```python
from build123d import *

# Parameters (mm, degrees)
ESBO_O1_R                = 1.393053459
ESBO_O1_R_2              = 4
ESBO_O1_R_3              = 1.370583382
RESSALTO_EXTRUS_O1_DEPTH = 40
CORTE_EXTRUS_O1_START    = -26
ESBO_O5_R                = 1.393053459
ESBO_O5_R_2              = 1.370583382
CORTE_EXTRUS_O1_DEPTH    = 26
ESBO_O8_W                = 7
ESBO_O8_H                = 2


with BuildPart() as part:
    # Esboço1 → Ressalto-extrusão1 (new body)
    with BuildSketch(Plane.XY):
        with BuildLine():
            Line((-90, -22.423877672), (-90, -19))
            ThreePointArc((-90, -19), (-71, 0), (-90, 19))
            Line((-90, 19), (-90, 23.042521341))
            Line((-90, 23.042521341), (-72.401791427, 23.042521341))
            ThreePointArc((-72.401791427, 23.042521341), (-59.673869366, 17.770443402), (-54.401791427, 5.042521341))
            Line((-54.401791427, 5.042521341), (-54.401791427, -4.423877672))
            ThreePointArc((-54.401791427, -4.423877672), (-59.673869366, -17.151799733), (-72.401791427, -22.423877672))
            Line((-72.401791427, -22.423877672), (-90, -22.423877672))
        make_face()
        with Locations((-64.399704634, 15.948259466)):
            Circle(ESBO_O1_R, mode=Mode.SUBTRACT)
        with Locations((-61.189365531, 0)):
            Circle(ESBO_O1_R_2, mode=Mode.SUBTRACT)
        with Locations((-64.399704634, -14.228928105)):
            Circle(ESBO_O1_R_3, mode=Mode.SUBTRACT)
    extrude(amount=RESSALTO_EXTRUS_O1_DEPTH)

    # Esboço5 → Corte-extrusão1 (cut)
    # profile 1 of 3: a face of its own
    with BuildSketch(Plane.XY.offset(40).offset(CORTE_EXTRUS_O1_START)):
        with BuildLine():
            add(Edge.make_bspline(
                [(-54.401791427, 5.042521341), (-55.530001159, 10.383788665), (-70.453859237, 8.636772089), (-68.317241022, 19.151967947), (-69.419494496, 22.655429754), (-72.401791427, 23.042521341)],
                knots=[0, 0, 0, 0, 0.59841234, 0.778329044, 1, 1, 1, 1], degree=3))
            ThreePointArc((-72.401791427, 23.042521341), (-59.673869366, 17.770443402), (-54.401791427, 5.042521341))
        make_face()
        with Locations((-64.399704634, 15.948259466)):
            Circle(ESBO_O5_R, mode=Mode.SUBTRACT)
    # profile 2 of 3: a face of its own
    with BuildSketch(Plane.XY.offset(40).offset(CORTE_EXTRUS_O1_START)):
        with BuildLine():
            add(Edge.make_bspline(
                [(-54.455116699, -5.808387052), (-55.021642733, -6.906023952), (-60.824639792, -8.65742119), (-69.99744996, -12.030398314), (-68.624992944, -17.552582132), (-68.947451642, -20.712215011), (-69.65151808, -21.847158712), (-70.29295532, -22.299917789)],
                knots=[0.054307943, 0.054307943, 0.054307943, 0.054307943, 0.303140082, 0.59841234, 0.778329044, 0.849345989, 0.932732603, 0.932732603, 0.932732603, 0.932732603], degree=3))
            ThreePointArc((-70.29295532, -22.299917789), (-59.419167454, -16.891895749), (-54.455116699, -5.808387052))
        make_face()
        with Locations((-64.399704634, -14.228928105)):
            Circle(ESBO_O5_R_2, mode=Mode.SUBTRACT)
    # profile 3 of 3: a face of its own
    with BuildSketch(Plane.XY.offset(40).offset(CORTE_EXTRUS_O1_START)):
        with Locations((-64.399704634, 15.948259466)):
            Circle(ESBO_O5_R)
    extrude(amount=CORTE_EXTRUS_O1_DEPTH, mode=Mode.SUBTRACT)

    # Varredura de corte1: sweep along a path in Esboço7
    with BuildLine(Plane.XY.offset(40)) as varredura_de_corte1_path:
        Line((-90, 23.042521341), (-72.401791427, 23.042521341))
        ThreePointArc((-72.401791427, 23.042521341), (-59.673869366, 17.770443402), (-54.401791427, 5.042521341))
        Line((-54.401791427, 5.042521341), (-54.401791427, -4.423877672))
        ThreePointArc((-54.401791427, -4.423877672), (-54.415127686, -5.116645636), (-54.455116699, -5.808387052))
        ThreePointArc((-54.455116699, -5.808387052), (-59.419167454, -16.891895749), (-70.29295532, -22.299917789))
        ThreePointArc((-70.29295532, -22.299917789), (-71.345553317, -22.392860978), (-72.401791427, -22.423877672))
        Line((-72.401791427, -22.423877672), (-90, -22.423877672))
    # Esboço8 → Varredura de corte1 (sweep, cut)
    with BuildSketch(Plane.ZY.offset(90)):
        with Locations((31.583750193, 22.042521341)):
            Rectangle(ESBO_O8_W, ESBO_O8_H)
        with Locations((14.959531016, 22.042521341)):
            Rectangle(ESBO_O8_W, ESBO_O8_H)
    sweep(path=varredura_de_corte1_path.line, mode=Mode.SUBTRACT)


solid = part.part
```
Check sheet for the modelled part. Datum: model origin and axes. Units: mm. A direction names the side the tool comes from. Coordinates: 2 decimals unless noted, no trailing zeros. Loops run counter-clockwise (first coordinate to the right, second up) from the corner with the lowest first, then second, coordinate; pieces in that order, holes last. Notation, with made-up numbers: M -21.5,-10 L 26.5,-10 A34 cw 26.5,28 Z; hole C -38,-11.75 d1. An arc over 180 degrees is marked long. Answer as a JSON object with one key per item and string values.
1. Sectioned sample at A-A on y = 0. Record the cut outline in (x, z), and give its area (3 significant figures).
Outcome:
{"outline": "M -71,0 L -65.19,0 L -65.19,40 L -71,40 Z; M -57.19,0 L -54.4,0 L -54.4,11.46 L -56.4,11.46 L -56.4,18.46 L -54.4,18.46 L -54.4,28.08 L -56.4,28.08 L -56.4,35.08 L -54.4,35.08 L -54.4,40 L -57.19,40 Z", "area": "316 mm²"}
2. Sectioned sample at B-B on x = -74. Record the cut outline in (y, z).
Outcome:
{"outline": "M -22.42,0 L -10.25,0 L -10.25,40 L -22.42,40 L -22.42,35.08 L -20.42,35.08 L -20.42,28.08 L -22.42,28.08 L -22.42,18.46 L -20.42,18.46 L -20.42,11.46 L -22.42,11.46 Z; M 10.25,0 L 23.04,0 L 23.04,11.46 L 21.04,11.46 L 21.04,18.46 L 23.04,18.46 L 23.04,28.08 L 21.04,28.08 L 21.04,35.08 L 23.04,35.08 L 23.04,40 L 10.25,40 Z"}
3. Depth check by flat-ended pin: P1, Ø5.5, axis at y = 1, z = 15, coming from the +X side; P2, Ø1.5, axis at y = 14.5, z = 30, coming from the +X side; P3, Ø3, axis at y = -6.5, z = 34.5, coming from the -X side. Enter the tip coordinate at first touch or a pass-through.
Outcome:
{"P1": "x = -56.4", "P2": "x = -68.73", "P3": "x = -72.77"}
4. Release check for a two-part mould opening along X. For faces 1 (the flat face through (-81, 21.043, 15)), 2 (the cylindrical face through (-65.77, -14.17, 6.9)), 3 (the flat face through (-90, 21, 20)) record: pulls with the +X half, pulls with the -X half, needs draft (parallel to the pull), parting line crosses it, or undercut.
Outcome:
{"face 1": "needs draft", "face 2": "undercut", "face 3": "pulls with the -X half"}
5. Scan lines: L1, parallel to Y at x = -64, z = 6.5; L2, parallel to Z at x = -62, y = -11; L3, parallel to Y at x = -79.5, z = 31.5. Record each from-to range of solid material in increasing order. Write a range as from..to.
Outcome:
{"L1": "-20.34..-15.54, -12.92..-2.85, 2.85..14.61, 17.28..20.96", "L2": "0..14", "L3": "-20.42..-15.84, 15.84..21.04"}
6. Access from +Z, -Z, +X, -X, +Y, -Y to the whole of each face (thin tool, end or side, straight path). Record for faces 4 (the flat face through (-55, 0, 11.46)), 5 (the flat face through (-81, 21.043, 32)), 6 (the flat face through (-81, -20.424, 32)).
Outcome:
{"face 4": "+X", "face 5": "+X, -X, +Y", "face 6": "+X, -X, -Y"}
